from build123d import *

# Parameters (mm, degrees)
SKETCH_1_R          = 11
EXTRUDE_1_DEPTH     = 17
SKETCH_2_R          = 9.582864225
CUT_EXTRUDE_1_DEPTH = 16
SKETCH_3_R          = 9.157454318
EXTRUDE_2_DEPTH     = 16


with BuildPart() as part:
    # 草图1 → 凸台-拉伸1 (new body)
    with BuildSketch(Plane(origin=(0, 0, 0), x_dir=(1, 0, 0), z_dir=(0, 1, 0))):
        with Locations(Location((0, 0, 0), (0, 0, 270))):
            Circle(SKETCH_1_R)
    extrude(amount=EXTRUDE_1_DEPTH)

    # 草图2 → 切除-拉伸1 (cut)
    with BuildSketch(Plane(origin=(0, 17, 0), x_dir=(1, 0, 0), z_dir=(0, 1, 0))):
        with Locations(Location((0, 0, 0), (0, 0, 270))):
            Circle(SKETCH_2_R)
    extrude(amount=-CUT_EXTRUDE_1_DEPTH, mode=Mode.SUBTRACT)

    # 草图3 → 凸台-拉伸2 (add)
    with BuildSketch(Plane(origin=(0, 1, 0), x_dir=(1, 0, 0), z_dir=(0, 1, 0))):
        with Locations(Location((0, 0, 0), (0, 0, 270))):
            Circle(SKETCH_3_R)
    extrude(amount=EXTRUDE_2_DEPTH)


solid = part.part
Geometry check sheet. Reference: the model listing, model coordinates, mm. Round coordinates to 2 decimals unless told otherwise and drop trailing zeros. Order: outer loops, then holes, each group sorted by start corner. A loop starts at its lowest first (then second) coordinate and runs counter-clockwise, first axis right, second up. Notation, with made-up numbers: M 56.5,68.25 L 85.5,68.25 A27 ccw 85.5,95.25 Z; hole C -3,-26.75 d2. An arc over 180 degrees is marked long. Answer in a Markdown table with one row per item. Add a question column.
Item 1: Sectioned sample at C-C, the plane x = 0. Enter the section's corners in (y, z).
Item 2: Sectioned sample at A-A, the plane y = 5.25. Enter the section's corners in (x, z), plus the area to 3 significant figures.
Item 3: Draft check along X on faces 1 (the face through (2.751, 8.888, 8.735)), 2 (the face through (-5.831, 9.112, -7.605)), 3 (the face through (-10.74, 8.38, -2.38)), 4 (the face through (0, 0, 0)). Enter one of: released by +X, released by -X, zero draft, split by the parting line, or undercut.
Item 4: Material ranges on L1, parallel to X at y = 8.25, z = 0; L2, parallel to Z at x = 0.25, y = 8.75; L3, parallel to Z at x = 7.5, y = 12.25 (3 decimals), recorded low to high. Write a range as [from, to].
Item 5: Depth check by flat-ended pin: pin 1 Ø2 at (y, z) = (15, 9) entering from +X; pin 2 Ø5 at (y, z) = (12, 3.5) entering from -X; pin 3 Ø1.5 at (x, y) = (7, 13.5) entering from +Z. Enter the tip coordinate at first touch or a pass-through.
Item 6: Sectioned sample at B-B, the plane z = 0. Enter the section's corners in (x, y).
Filled in:
| question | item | result |
|---|---|---|
| 1 | outline | M 0,-11 L 17,-11 L 17,-9.58 L 1,-9.58 L 1,-9.16 L 17,-9.16 L 17,9.16 L 1,9.16 L 1,9.58 L 17,9.58 L 17,11 L 0,11 Z |
| 2 | outline | C 0,0 d22; C 0,0 d18.31; hole C 0,0 d19.17 |
| 2 | area | 355 mm² |
| 3 | face 1 | undercut |
| 3 | face 2 | undercut |
| 3 | face 3 | split by the parting line |
| 3 | face 4 | zero draft |
| 4 | L1 | x = [-11, -9.58], [-9.16, 9.16], [9.58, 11] |
| 4 | L2 | z = [-11, -9.58], [-9.15, 9.15], [9.58, 11] |
| 4 | L3 | z = [-8.047, -5.965], [-5.254, 5.254], [5.965, 8.047] |
| 5 | pin 1 | stops at x = 7.55 |
| 5 | pin 2 | stops at x = -10.95 |
| 5 | pin 3 | stops at z = 9.05 |
| 6 | outline | M -11,0 L 11,0 L 11,17 L 9.58,17 L 9.58,1 L 9.16,1 L 9.16,17 L -9.16,17 L -9.16,1 L -9.58,1 L -9.58,17 L -11,17 Z |
